Autodesk Fusion 360 part; units mm, degrees
sketch "Sketch1" plane through (0, 0, 0) normal (0, 1, 0) x (1, 0, 0)
  line L0 (18, 10.75) -> (-18, 10.75)
  line L1 (-20, 8.75) -> (-20, -10.75)
  line L2 (-20, -10.75) -> (20, -10.75)
  line L3 (20, -10.75) -> (20, 8.75)
  line L4 (20, 10.75) -> (-20, -10.75) construction
  line L5 (-20, 10.75) -> (20, -10.75) construction
  arc A0 (-18, 10.75) -> (-20, 8.75) centre (-18, 8.75) ccw
  arc A1 (20, 8.75) -> (18, 10.75) centre (18, 8.75) ccw
  dimension "d1" = 40
  dimension "d2" = 21.5
  dimension "d3" = 2
extrude "Extrude1" add sketch "Sketch1" along normal blind 1.5
sketch "Sketch2" plane through (0, 0, 10.75) normal (0, 0, 1) x (1, 0, 0)
  line L0 (-20, 0) -> (20, 0)
  line L1 (20, 0) -> (20, 1.5)
  line L2 (20, 1.5) -> (-20, 1.5)
  line L3 (-20, 1.5) -> (-20, 0)
  line L4 (-20, 1.5) -> (20, 1.5)
  line L5 (20, 1.5) -> (20, -34)
  line L6 (15, -39) -> (-15, -39)
  line L7 (-20, -34) -> (-20, 1.5)
  circle A0 centre (0, -18.75) radius 7
  arc A1 (-20, -34) -> (-15, -39) centre (-15, -34) ccw
  arc A2 (15, -39) -> (20, -34) centre (15, -34) ccw
  point P0 (-20, -39)
  dimension "d7" = 40.5
  dimension "d8" = 14
  dimension "d11" = 5
extrude "Extrude2" add sketch "Sketch2" against normal blind 1.5
Model file for the job. Use its own axes, mm. A direction names the side the tool comes from. Round coordinates to 2 decimals unless told otherwise and drop trailing zeros. Order: outer loops, then holes, each group sorted by start corner. A loop starts at its lowest first (then second) coordinate and runs counter-clockwise, first axis right, second up. Notation, with made-up numbers: M -21.75,50.5 L 29.25,50.5 A23 cw 29.25,83.5 Z; hole C 75.25,33.5 d1. An arc over 180 degrees is marked long. Write each question's results on one line, items separated by ' | '. Start each with the question number.
(1) Which spindle directions (+Z, -Z, +X, -X, +Y, -Y) get a long thin tool onto all of the face, cutting with end or side? Do faces 5 (the face through (-19, -37, 10)), 6 (the face through (0, -28, 9.25)). Say none if no direction does.
(2) Saw through at C-C, the plane x = 11. Give the cut face in (y, z).
(3) Two-plate mould, pull along Y, no slides. Class faces 1 (the face through (9, -19, 10.75)), 2 (the face through (0, -39, 10)), 3 (the face through (0, 1.5, 0)), 4 (the face through (-1.517, -25.584, 10.01)): pulls with the +Y half, pulls with the -Y half, needs draft (parallel to the pull), parting line crosses it, or undercut.
(4) Saw through at B-B, the plane x = 0. Give the cut face in (y, z), then the cut area to 4 significant figures.
(5) Saw through at A-A, the plane y = -18.75. Give the cut face in (x, z).
(6) Probe probe 1 along Y at (x, z) = (0, 9.75); probe 2 along Z at (x, y) = (9, -27); probe 3 along Y at (x, z) = (3.5, 3). List the from-to ranges inside material, lowest first. Write a range as from..to.
(7) Saw through at D-D, the plane z = -1.25. Give the cut face in (x, y), then the cut area to 3 significant figures.
(8) Drop flat-ended pins along their axis: pin 1 (1 mm diameter, centred on x = 13.5, y = -21.5, fed in from -Z); pin 2 (6 mm diameter, centred on x = 3, z = 0, fed in from -Y). Give the stop position or say it passes through.
Established:
1) face 5: +Z, -Z, -X, -Y | face 6: -Z, +X, -X, -Y
2) outline: M -39,9.25 L 0,9.25 L 0,-10.75 L 1.5,-10.75 L 1.5,10.75 L -39,10.75 Z
3) face 1: needs draft | face 2: pulls with the -Y half | face 3: pulls with the +Y half | face 4: undercut
4) outline: M -39,9.25 L -25.75,9.25 L -25.75,10.75 L -39,10.75 Z; M -11.75,9.25 L 0,9.25 L 0,-10.75 L 1.5,-10.75 L 1.5,10.75 L -11.75,10.75 Z | area: 69.75 mm^2
5) outline: M -20,9.25 L -7,9.25 L -7,10.75 L -20,10.75 Z; M 7,9.25 L 20,9.25 L 20,10.75 L 7,10.75 Z
6) probe 1: y = -39..-25.75, -11.75..1.5 | probe 2: z = 9.25..10.75 | probe 3: y = 0..1.5
7) outline: M -20,0 L 20,0 L 20,1.5 L -20,1.5 Z | area: 60.0 mm^2
8) pin 1: stops at z = 9.25 | pin 2: stops at y = 0
